Input: dimensioned drawing with shaded views. Units: mm. Origin: part minimum x, y, z. Coordinates: 2 decimals unless noted, no trailing zeros. Loops run counter-clockwise (first coordinate to the right, second up) from the corner with the lowest first, then second, coordinate; pieces in that order, holes last.
Item 1: Pin query (flat end, axial travel): pin 1 Ø2.5 at (x, y) = (5, 15) entering from -Z; pin 2 Ø3 at (x, y) = (5, 3) entering from -Z. Return the tip coordinate at first contact, or that it passes through.
Item 2: Section query B-B, the plane y = 5. Return the cut outline in (x, z), then the cut area to 3 significant figures.
Item 3: Section query D-D, the plane y = 15.75. Return the cut outline in (x, z).
Item 4: Section query A-A, the plane x = 5. Return the cut outline in (y, z), then the cut area to 3 significant figures.
Item 5: Pull-direction query (X, two-part tool) for the marked faces 1, 2 and 3; classes: +X half, -X half, draft (parallel to the pull), parting line (faces both ways), or undercut.
Item 6: Section query C-C, the plane z = 1.3. Return the cut outline in (x, y).
Item 7: Line query: probe 1 along Y at (x, z) = (5, 0.4); probe 2 along X at (y, z) = (15.25, 1.75); probe 3 along X at (y, z) = (16, 0.75). Output: solid intervals per line, ascending.
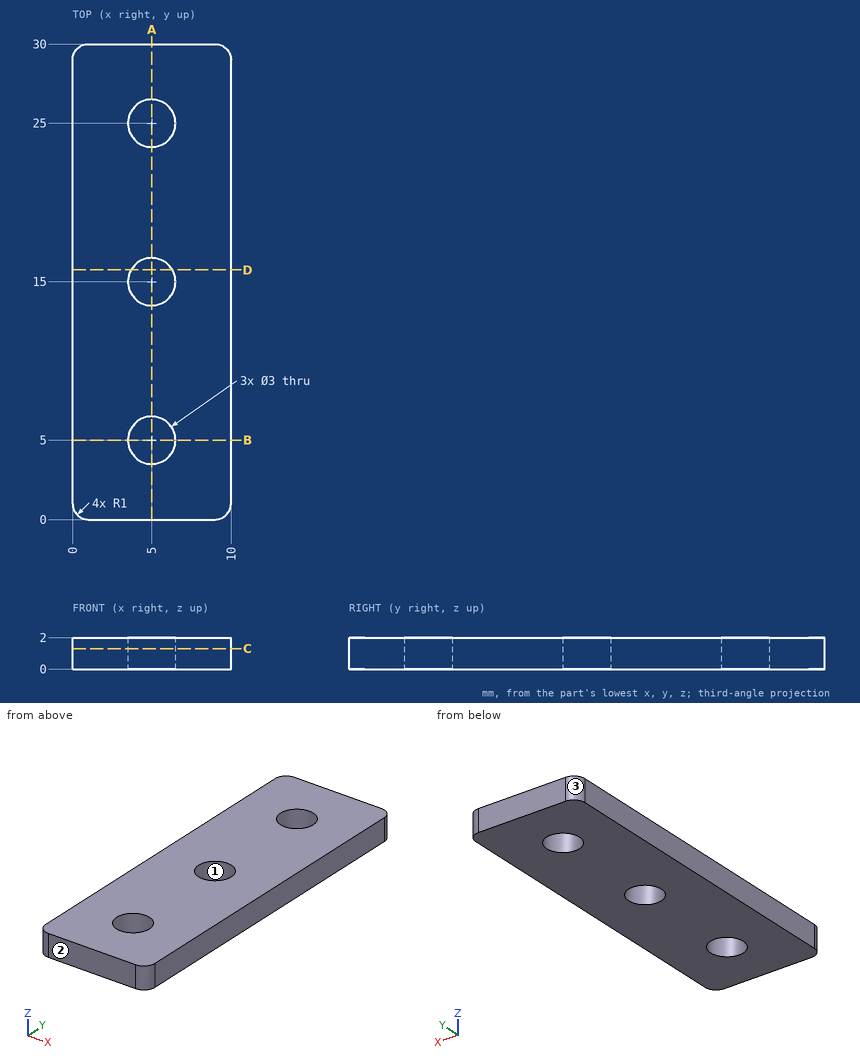
Verdict:
1. pin 1: passes through
1. pin 2: stops at z = 0
2. outline: (0, 0) - (3.5, 0) - (3.5, 2) - (0, 2) - close; (6.5, 0) - (10, 0) - (10, 2) - (6.5, 2) - close
2. area: 14.0 mm2
3. outline: (0, 0) - (3.7, 0) - (3.7, 2) - (0, 2) - close; (6.3, 0) - (10, 0) - (10, 2) - (6.3, 2) - close
4. outline: (0, 0) - (3.5, 0) - (3.5, 2) - (0, 2) - close; (6.5, 0) - (13.5, 0) - (13.5, 2) - (6.5, 2) - close; (16.5, 0) - (23.5, 0) - (23.5, 2) - (16.5, 2) - close; (26.5, 0) - (30, 0) - (30, 2) - (26.5, 2) - close
4. area: 42.0 mm2
5. face 1: undercut
5. face 2: draft
5. face 3: -X half
6. outline: (0, 1) arc R1 ccw to (1, 0) - (9, 0) arc R1 ccw to (10, 1) - (10, 29) arc R1 ccw to (9, 30) - (1, 30) arc R1 ccw to (0, 29) - close; hole circle Ø3 at (5, 5); hole circle Ø3 at (5, 15); hole circle Ø3 at (5, 25)
7. probe 1: y = 0 to 3.5, 6.5 to 13.5, 16.5 to 23.5, 26.5 to 30
7. probe 2: x = 0 to 3.52, 6.48 to 10
7. probe 3: x = 0 to 3.88, 6.12 to 10
